Autodesk Inventor part; units mm, degrees
ref_plane "YZ Plane" through (0, 0, 0) normal (1, 0, 0) x (0, 1, 0)
ref_plane "XZ Plane" through (0, 0, 0) normal (0, 1, 0) x (-1, 0, 0)
ref_plane "XY Plane" through (0, 0, 0) normal (0, 0, 1) x (1, 0, 0)
ref_plane "Plano de trabalho1" through (0, 0, 0) normal (0, 0, 1) x (1, 0, 0)
sketch "Esboço1" plane through (0, 0, 0) normal (0, 0, 1) x (1, 0, 0)
  arc A0 (-40.8144, 85.0081) -> (-13.8144, 85.0195) centre (-27.3144, 85.0138) ccw
  circle A1 centre (-27.3144, 85.0138) radius 13.5
  line L0 (-40.8144, 85.0081) -> (-45.8144, 85.006)
  line L1 (-45.8144, 85.006) -> (-55.8144, 85.0017)
  line L2 (-55.8144, 85.0017) -> (-13.8144, 85.0195)
  line L3 (-13.8144, 85.0195) -> (-8.8144, 85.0216)
  line L4 (-8.8144, 85.0216) -> (1.1856, 85.0259)
  line L5 (1.1856, 85.0259) -> (1.1834, 90.0259)
  line L6 (1.1834, 90.0259) -> (-14.7766, 90.0191)
  line L7 (-55.8144, 85.0017) -> (-55.8166, 90.0017)
  line L8 (-55.8166, 90.0017) -> (-39.8565, 90.0085)
  line L9 (-27.3144, 98.5138) -> (-27.3166, 103.5138)
  arc A2 (-8.8144, 85.0216) -> (-45.8144, 85.006) centre (-27.3144, 85.0138) ccw
  point P0 (0, 0)
  point P1 (-40.8144, 85.0081)
  point P2 (-13.8144, 85.0195)
  point P3 (-9.5051, 90.0213)
  point P4 (-45.1281, 90.0062)
  dimension "d0" = 27
  dimension "d1" = 13.5
  dimension "d2" = 5
  dimension "d3" = 10
  dimension "d4" = 5
  dimension "d5" = 10
  dimension "d6" = 5
  dimension "d7" = 5
  dimension "d8" = 5
extrude "Extrusão1" add sketch "Esboço1" against normal blind 20 contours L0 A2 L8 A1 | L8 A2 L9 A1 | L1 L7 L8 A2 | A1 L6 A2 L3 | L9 A2 L6 A1 | A2 L6 L5 L4
fillet "Arredondamento1" radius 6 4 edges at (1.1845, 87.5259, 0) (1.1845, 87.5259, -20) (-55.8155, 87.5017, 0) (-55.8155, 87.5017, -20)
sketch "Esboço2" plane through (-13.8144, 85.0195, -20) normal (0.0004, -1, 0) x (1, 0.0004, 0)
  arc A0 (9.2495, 14.6999) -> (10.7509, 14.6999) centre (10.0003, 16.0018) ccw
  circle A1 centre (10.0003, 16.0018) radius 1.5029
  arc A2 (9.2495, 2.6941) -> (10.7509, 2.6875) centre (10.0061, 4.0358) ccw
  circle A3 centre (10.0061, 4.0358) radius 1.5402
  arc A4 (-37.7345, 14.6999) -> (-36.2329, 14.6999) centre (-36.9837, 16.0022) ccw
  circle A5 centre (-36.9837, 16.0022) radius 1.5032
  line L0 (-36.2329, 2.6941) -> (-37.7345, 2.6941)
  line L1 (-37.7345, 2.6941) -> (-36.2546, 4.1926)
  arc A6 (-37.7345, 2.6941) -> (-36.2329, 2.6941) centre (-36.9837, 4.0136) ccw
  circle A7 centre (-36.9837, 4.0136) radius 1.5181
  point P0 (13.7784, 20)
  point P1 (10.7509, 2.6875)
  point P2 (9.2495, 2.6941)
  point P3 (10.7509, 14.6999)
  point P4 (9.2495, 14.6999)
  point P5 (-36.2329, 14.6999)
  point P6 (-37.7345, 14.6999)
  point P7 (-37.7345, 2.6941)
  point P8 (-36.2329, 2.6941)
extrude "Extrusão2" cut sketch "Esboço2" against normal blind 20
properties part number "Capa suporte"
The listing builds one solid part. Answer for the finished solid, in the listing's coordinates (mm). Give positions to 0.01 mm unless a question says otherwise; leave off trailing zeros. Order: outer loops, then holes, each group sorted by start corner. A loop starts at its lowest first (then second) coordinate and runs counter-clockwise, first axis right, second up. Notation, with made-up numbers: M 76.25,85 L 91.25,85 A17 cw 91.25,97 Z; hole C 55,-35 d5. An arc over 180 degrees is marked long. Put each result on its own line as item: value. Start each with the question number.
Item 1: The part is cut by section C-C, the plane z = -7. Determine the outline of the cut face in (x, y) (1 decimal).
Item 2: Flat-ended cylindrical pins translate along their axes: P1, Ø3, axis at y = 100.5, z = -15.5, coming from the -X side; P2, Ø5.5, axis at x = -49, z = -11, coming from the +Y side; P3, Ø1, axis at x = -23.5, z = -13.5, coming from the +Y side. Find the tip coordinate at first contact, or state that the pin passes through.
Item 3: The part is cut by section A-A, the plane z = -4. Determine the outline of the cut face in (x, y) (1 decimal), and give its area (3 significant figures).
Item 4: The part is cut by section B-B, the plane y = 93.5. Determine the outline of the cut face in (x, z), and give its area (3 significant figures).
Item 5: The part is cut by section D-D, the plane y = 87.5. State how many separate pieces and enclosed holes the cut face has, and give its area (3 significant figures).
Item 6: Find the intervals of material crossed by line 1 along Y through (x, z) = (-52, -17.5); line 2 along X through (y, z) = (91, -13.5); line 3 along X through (y, z) = (87.5, -9.75), in increasing order.
Item 7: For a pull along Z with two mould halves and no side action, classify faces 1 (the face through (-27, 100, 0)), 2 (the face through (-26.99, 103.51, -9.86)), 3 (the face through (-3.746, 87.489, -14.425)) as +Z half, -Z half, draft (parallel to the pull), parting line (faces both ways), or undercut.
Answer key:
1. outline: M -55.8,85 L -45.8,85 L -40.8,85 A13.5 cw -13.8,85 L -8.8,85 L 1.2,85 L 1.2,90 L -9.5,90 A18.5 ccw -45.1,90 L -55.8,90 Z
2. P1: stops at x = -39.42
2. P2: stops at y = 90.01
2. P3: stops at y = 103.21
3. outline: M -55.5,85 L -52.3,85 L -52.3,90 L -55.5,90 Z; M -49.3,85 L -45.8,85 L -40.8,85 A13.5 cw -13.8,85 L -8.8,85 L -5.3,85 L -5.3,90 L -9.5,90 A18.5 ccw -45.1,90 L -49.3,90 Z; M -2.3,85 L 0.8,85 L 0.8,90 L -2.3,90 Z
3. area: 320 mm²
4. outline: M -43.75,-20 L -37.81,-20 L -37.81,0 L -43.75,0 Z; M -16.82,-20 L -10.88,-20 L -10.88,0 L -16.82,0 Z
4. area: 238 mm²
5. separate pieces: 2
5. enclosed holes: 4
5. area: 549 mm²
6. line 1: y = 85 to 90
6. line 2: x = -44.82 to -39.41, -15.21 to -9.81
6. line 3: x = -55.82 to -40.58, -14.05 to 1.18
7. face 1: +Z half
7. face 2: draft
7. face 3: undercut
